from build123d import *

# Parameters (mm, degrees)
MAIN_BOBY_DEPTH                                 = 40
WALL_THICKNESS_T                                = -6
RIB_DEPTH                                       = 21.5
TOP_BOSS_DEPTH                                  = 25
TABS_DEPTH                                      = 20
V_SLOT_DEPTH                                    = 103.5
V_SLOT_DEPTH_BACK                               = 103.5
U_CUTOUT_REACH                                  = 127
BOTTOM_BOSS_DEPTH                               = 25
LARGE_HOLES_REACH                               = 33
SKETCH8_R                                       = 12.7
CSK_FOR_M6_FLAT_HEAD_MACHINE_SCREW1_D           = 6.6
CSK_FOR_M6_FLAT_HEAD_MACHINE_SCREW1_CSINK_D     = 12.6
CSK_FOR_M6_FLAT_HEAD_MACHINE_SCREW1_CSINK_ANGLE = 90
CBORE_FOR_M8_SHCS1_D                            = 9
CBORE_FOR_M8_SHCS1_DEPTH                        = 25
CBORE_FOR_M8_SHCS1_CBORE_D                      = 15
CBORE_FOR_M8_SHCS1_CBORE_DEPTH                  = 8
M6X1_0_TAPPED_HOLE1_D                           = 5
M6X1_0_TAPPED_HOLE1_DEPTH                       = 17
M6X1_0_TAPPED_HOLE1_TIP                         = 1.502151548
M8X1_25_TAPPED_HOLE2_D                          = 6.8
M8X1_25_TAPPED_HOLE2_DEPTH                      = 20
FILLET1_R                                       = 6
CHAMFER1_SIZE                                   = 10
CHAMFER2_SIZE                                   = 6


with BuildPart() as part:
    # Sketch1 → Main Boby (new body)
    with BuildSketch(Plane.XY):
        Polygon((80, 200), (-80, 200), (-45, 0), (45, 0), align=None)
    extrude(amount=MAIN_BOBY_DEPTH)

    # Wall Thickness
    wall_thickness_openings = [part.faces().sort_by_distance(p)[0] for p in [
        (0, 100, 40),
    ]]
    offset(amount=WALL_THICKNESS_T, openings=wall_thickness_openings, kind=Kind.INTERSECTION)

    # Sketch2 → Rib (add)
    with BuildSketch(Plane.XY.offset(6)):
        Polygon((-66.875, 125), (-25, 125), (-25, 100), (25, 100), (25, 125), (66.875, 125), (66.875, 128.5), (21.5, 128.5), (21.5, 103.5), (-21.5, 103.5), (-21.5, 128.5), (-66.875, 128.5), align=None)
    extrude(amount=RIB_DEPTH)

    # Sketch3 → Top Boss (add)
    with BuildSketch(Plane(origin=(0, 0, 0), x_dir=(-1, 0, 0), z_dir=(0, 0, -1))):
        Polygon((-84.375, 225), (84.375, 225), (75.625, 175), (-75.625, 175), align=None)
    extrude(amount=TOP_BOSS_DEPTH)

    # Sketch4 → Tabs (add)
    with BuildSketch(Plane.XY.offset(40)):
        with BuildLine():
            Line((80, 200), (92.5, 200))
            ThreePointArc((92.5, 200), (102.5, 190), (92.5, 180))
            Line((92.5, 180), (76.5, 180))
            Line((76.5, 180), (80, 200))
        make_face()
        with BuildLine():
            Line((64.25, 110), (76.75, 110))
            ThreePointArc((76.75, 110), (86.75, 100), (76.75, 90))
            Line((76.75, 90), (60.75, 90))
            Line((60.75, 90), (64.25, 110))
        make_face()
        with BuildLine():
            Line((48.5, 20), (61, 20))
            ThreePointArc((61, 20), (71, 10), (61, 0))
            Line((61, 0), (45, 0))
            Line((45, 0), (48.5, 20))
        make_face()
    tabs = extrude(amount=-TABS_DEPTH)

    # Mirror1: Tabs across plane
    add(tabs.mirror(Plane(origin=(0, 0, 0), x_dir=(0, 0, 1), z_dir=(1, 0, 0))))

    # Sketch5 → V Slot (cut, two sides)
    with BuildSketch(Plane(origin=(0, 0, 0), x_dir=(0, 0, -1), z_dir=(1, 0, 0))) as v_slot_sk:
        Polygon((25, 212.5), (17.67766953, 212.5), (12.5, 200), (17.67766953, 187.5), (25, 187.5), align=None)
    extrude(amount=V_SLOT_DEPTH, mode=Mode.SUBTRACT)
    extrude(v_slot_sk.sketch, amount=-V_SLOT_DEPTH_BACK, mode=Mode.SUBTRACT)

    # Sketch6 → U Cutout (cut, up to next)
    with BuildSketch(Plane.XZ.offset(-100), mode=Mode.PRIVATE) as u_cutout_sk1:
        with BuildLine():
            Line((-6.25, 27.5), (-6.25, 17.5))
            ThreePointArc((-6.25, 17.5), (0, 11.25), (6.25, 17.5))
            Line((6.25, 17.5), (6.25, 27.5))
            Line((6.25, 27.5), (-6.25, 27.5))
        make_face()
    u_cutout_tool1 = extrude(u_cutout_sk1.sketch, amount=-U_CUTOUT_REACH, mode=Mode.PRIVATE) & part.part
    add(u_cutout_tool1.solids().sort_by_distance((0, 100, 19.980369))[0], mode=Mode.SUBTRACT)

    # Sketch7 → Bottom Boss (add)
    with BuildSketch(Plane(origin=(0, 0, 0), x_dir=(-1, 0, 0), z_dir=(0, 0, -1))):
        with BuildLine():
            Line((-12.5, 0), (-12.5, -25))
            ThreePointArc((-12.5, -25), (0, -37.5), (12.5, -25))
            Line((12.5, -25), (12.5, 0))
            Line((12.5, 0), (-12.5, 0))
        make_face()
    extrude(amount=-BOTTOM_BOSS_DEPTH)

    # Sketch8 → Large Holes (cut, up to next)
    with BuildSketch(Plane.XY.offset(6), mode=Mode.PRIVATE) as large_holes_sk1:
        with Locations((-37.5, 150)):
            Circle(SKETCH8_R)
    large_holes_tool1 = extrude(large_holes_sk1.sketch, amount=-LARGE_HOLES_REACH, mode=Mode.PRIVATE) & part.part
    add(large_holes_tool1.solids().sort_by_distance((-37.5, 150, 6))[0], mode=Mode.SUBTRACT)
    # Sketch8 → Large Holes (cut, up to next)
    with BuildSketch(Plane.XY.offset(6), mode=Mode.PRIVATE) as large_holes_sk2:
        with Locations((37.5, 150)):
            Circle(SKETCH8_R)
    large_holes_tool2 = extrude(large_holes_sk2.sketch, amount=-LARGE_HOLES_REACH, mode=Mode.PRIVATE) & part.part
    add(large_holes_tool2.solids().sort_by_distance((37.5, 150, 6))[0], mode=Mode.SUBTRACT)

    # CSK for M6 Flat Head Machine Screw1 (through all)
    with Locations(Plane.XY.offset(6)):
        with Locations((-25, 75), (25, 75), (25, 25), (-25, 25)):
            CounterSinkHole(CSK_FOR_M6_FLAT_HEAD_MACHINE_SCREW1_D / 2, CSK_FOR_M6_FLAT_HEAD_MACHINE_SCREW1_CSINK_D / 2, counter_sink_angle=CSK_FOR_M6_FLAT_HEAD_MACHINE_SCREW1_CSINK_ANGLE)

    # CBORE for M8 SHCS1
    with Locations(Plane.XY.offset(25)):
        with Locations((0, -25)):
            CounterBoreHole(CBORE_FOR_M8_SHCS1_D / 2, CBORE_FOR_M8_SHCS1_CBORE_D / 2, CBORE_FOR_M8_SHCS1_CBORE_DEPTH, depth=CBORE_FOR_M8_SHCS1_DEPTH)

    # M6x1.0 Tapped Hole1
    with Locations(Plane(origin=(0, 0, -25), x_dir=(-1, 0, 0), z_dir=(0, 0, -1))):
        with Locations((-62.5, 218.75), (0, 218.75), (62.5, 218.75)):
            Hole(M6X1_0_TAPPED_HOLE1_D / 2, depth=M6X1_0_TAPPED_HOLE1_DEPTH)
            with Locations((0, 0, -(M6X1_0_TAPPED_HOLE1_DEPTH + M6X1_0_TAPPED_HOLE1_TIP / 2))):  # 118° drill point
                Cone(0, M6X1_0_TAPPED_HOLE1_D / 2, M6X1_0_TAPPED_HOLE1_TIP, mode=Mode.SUBTRACT)

    # M8x1.25 Tapped Hole2
    with Locations(Plane.XY.offset(40)):
        with Locations((-92.5, 190), (92.5, 190), (76.75, 100), (-76.75, 100), (-61, 10), (61, 10)):
            Hole(M8X1_25_TAPPED_HOLE2_D / 2, depth=M8X1_25_TAPPED_HOLE2_DEPTH)

    # Fillet1
    fillet1_edges = [part.edges().sort_by_distance(p)[0] for p in [
        (48.5, 20, 30),
        (-76.5, 180, 30),
        (-64.25, 110, 30),
        (-60.75, 90, 30),
        (-48.5, 20, 30),
        (39.958817849, 6, 23),
        (72.858817849, 194, 23),
        (-72.858817849, 194, 23),
        (-39.958817849, 6, 23),
        (12.5, 0, 12.5),
        (-12.5, 0, 12.5),
        (60.783817849, 125, 16.75),
        (-60.783817849, 125, 16.75),
        (25, 125, 16.75),
        (61.396317849, 128.5, 16.75),
        (21.5, 103.5, 16.75),
        (-21.5, 103.5, 16.75),
        (-61.396317849, 128.5, 16.75),
        (-25, 125, 16.75),
        (76.5, 180, 30),
        (60.75, 90, 30),
        (64.25, 110, 30),
    ]]
    fillet(fillet1_edges, radius=FILLET1_R)

    # Chamfer1
    chamfer1_edges = [part.edges().sort_by_distance(p)[0] for p in [
        (0, 200, 0),
    ]]
    chamfer(chamfer1_edges, length=CHAMFER1_SIZE)

    # Chamfer2
    chamfer2_edges = [part.edges().sort_by_distance(p)[0] for p in [
        (21.5, 128.5, 16.75),
        (-21.5, 128.5, 16.75),
        (-25, 100, 16.75),
        (25, 100, 16.75),
    ]]
    chamfer(chamfer2_edges, length=CHAMFER2_SIZE)


solid = part.part
Can you work these out from the model? Positions are in its coordinate system, mm. A direction names the side the tool comes from. Give positions to 0.01 mm unless a question says otherwise; leave off trailing zeros. Loops run counter-clockwise (first coordinate to the right, second up) from the corner with the lowest first, then second, coordinate; pieces in that order, holes last. Notation, with made-up numbers: (83.25, -2) -> (124.25, -2) arc R28 cw to (124.25, 16) -> close; hole circle Ø4 at (76.5, 56). An arc over 180 degrees is marked (long way). Use one line per item in the form item = value.
1) We'd pull the mould along X, two halves only. Please class faces 1 (the face through (-12.5, -16, 12)), 2 (the face through (-25, 126, 17)), 3 (the face through (-1, 181, -25)): released by +X, released by -X, zero draft, split by the parting line, or undercut.
Answers:
face_1 = released by -X
face_2 = undercut
face_3 = zero draft
2) If we section it at B-B (y = 93): Please give me the cut outline in (x, z) (3 decimals).
Answers:
outline = (-83.891, 20) -> (-61.275, 20) -> (-61.275, 0) -> (61.275, 0) -> (61.275, 20) -> (83.891, 20) -> (83.891, 40) -> (55.184, 40) -> (55.184, 6) -> (-55.184, 6) -> (-55.184, 40) -> (-83.891, 40) -> close
3) Will these pins go through, and if not, where does the flat tip stop? pin 1 (9.5 mm diameter, centred on y = -14.5, z = 10.5, fed in from -X); pin 2 (12.5 mm diameter, centred on x = -86.5, y = 187.5, fed in from -Z); pin 3 (6 mm diameter, centred on x = 27.5, y = 86, fed in from -Z); pin 4 (8 mm diameter, centred on x = -62.5, y = 218.75, fed in from -Z).
Answers:
pin_1 = -12.5
pin_2 = 20
pin_3 = 0
pin_4 = -25
4) If we section it at A-A (y = 150): Please give me the cut outline in (x, z).
Answers:
outline = (-71.25, 0) -> (-50.2, 0) -> (-50.2, 6) -> (-65.16, 6) -> (-65.16, 40) -> (-71.25, 40) -> close; (-24.8, 0) -> (24.8, 0) -> (24.8, 6) -> (-24.8, 6) -> close; (50.2, 0) -> (71.25, 0) -> (71.25, 40) -> (65.16, 40) -> (65.16, 6) -> (50.2, 6) -> close
5) I need wall thicknesses on line 1 along Y through (x, z) = (-62, -19); line 2 along Y through (x, z) = (8, -21.5); line 3 along Y through (x, z) = (92.5, 28.5). Which ranges of each line are inside material? Lowest first, please.
Answers:
line_1 = 175 to 187.5, 212.5 to 216.3, 221.2 to 225
line_2 = 175 to 187.5, 212.5 to 225
line_3 = 180 to 186.6, 193.4 to 200
6) For faces 4 (the face through (64.41, 110.92, 15.18)), 5 (the face through (-74, 110, 30)), 6 (the face through (87, 180, 30)), which set-ups out of +Z, -Z, +X, -X, +Y, -Y let a thin tool reach every point of the face, with its end or its side?
Answers:
face_4 = -Z, +X
face_5 = +Z, -Z, -X
face_6 = +Z, -Z, +X
